from build123d import *

# Parameters (mm, degrees)
BOSS_EXTRUDE1_DEPTH = 5.9944
CUT_EXTRUDE2_REACH  = 7.994


with BuildPart() as part:
    # Sketch1 → Boss-Extrude1 (new body)
    with BuildSketch(Plane.XY):
        Polygon((-3.048, 63.5), (-3.048, 127), (0, 127), (0, 190.5), (-3.048, 190.5), (-3.048, 253.981711342), (59.0804, 253.981711342), (59.0804, 248.012711342), (118.1608, 248.012711342), (118.1608, 253.981711342), (177.2412, 253.981711342), (177.2412, 248.012711342), (236.3216, 248.012711342), (236.3216, 253.981711342), (295.402, 253.981711342), (295.402, 190.481711342), (298.45, 190.481711342), (298.45, 126.981711342), (295.402, 126.981711342), (295.402, 63.5), (298.45, 63.5), (298.45, 0), (0, 0), (0, 63.5), align=None)
    extrude(amount=BOSS_EXTRUDE1_DEPTH)

    # Sketch2 → Cut-Extrude2 (cut, up to next)
    with BuildSketch(Plane.XY.offset(5.9944), mode=Mode.PRIVATE) as cut_extrude2_sk1:
        with BuildLine():
            Line((270.51, 2.54), (270.51, 0))
            Line((270.51, 0), (275.59, 0))
            Line((275.59, 0), (275.59, 2.54))
            ThreePointArc((275.59, 2.54), (273.05, 5.08), (270.51, 2.54))
        make_face()
    cut_extrude2_tool1 = extrude(cut_extrude2_sk1.sketch, amount=-CUT_EXTRUDE2_REACH, mode=Mode.PRIVATE) & part.part
    add(cut_extrude2_tool1.solids().sort_by_distance((273.05, 2.302891, 5.9944))[0], mode=Mode.SUBTRACT)


solid = part.part
The listing builds one solid part. Answer for the finished solid, in the listing's coordinates (mm). A direction names the side the tool comes from. Coordinates: 2 decimals unless noted, no trailing zeros. Write each loop counter-clockwise with the first axis right and the second up, starting at its lowest first coordinate (ties: lowest second). Pieces come first, ordered by that corner, then holes. Notation, with made-up numbers: M 25,13.25 L 51,13.25 A16 cw 51,25.25 Z; hole C 23,71.5 d8. An arc over 180 degrees is marked long. Put each result on its own line as item: value. Start each with the question number.
1. Consider line 1 (X direction, y = 221, z = 1); line 2 (X direction, y = 187.5, z = 2.25); line 3 (Y direction, x = 273, z = 5.45). Determine where each line is inside the solid, lowest interval first. Write a range as from..to.
2. Which of the six approach directions +Z, -Z, +X, -X, +Y, -Y give full straight-line access (tool end or side, diameter ignored) to faces 1 (the flat face through (0, 31, 3)), 2 (the flat face through (0, 158, 3)), 3 (the flat face through (88, 248.013, 3)), 4 (the flat face through (295.402, 223, 3))?
3. A cutting plane is placed at A-A on z = 3.35. Write down the section's boundary in (x, y), then the cut area to 3 significant figures.
4. For a pull along X with two mould halves and no side action, classify faces 5 (the flat face through (298.45, 159, 3)), 6 (the flat face through (59.08, 251, 3)), 7 (the flat face through (287, 0, 3)) as pulls with the +X half, pulls with the -X half, needs draft (parallel to the pull), parting line crosses it, or undercut.
5. A cutting plane is placed at B-B on x = 195. Write down the section's boundary in (y, z).
6. Flat-ended cylindrical pins translate along their axes: P1, Ø1.5, axis at x = 297.5, z = 4, coming from the +Y side; P2, Ø3, axis at y = 232, z = 2.5, coming from the +X side; P3, Ø3.5, axis at x = -1.5, z = 4.5, coming from the -Y side; P4, Ø3, axis at y = 1.5, z = 2, coming from the -X side. Find the tip coordinate at first contact, or state that the pin passes through.
Resolved:
1. line 1: x = -3.05..295.4
1. line 2: x = 0..298.45
1. line 3: y = 5.08..253.98
2. face 1: +Z, -Z, -X, -Y
2. face 2: +Z, -Z, -X
2. face 3: +Z, -Z, +Y
2. face 4: +Z, -Z, +X, +Y
3. outline: M -3.05,63.5 L 0,63.5 L 0,0 L 270.51,0 L 270.51,2.54 A2.54 cw 275.59,2.54 L 275.59,0 L 298.45,0 L 298.45,63.5 L 295.4,63.5 L 295.4,126.98 L 298.45,126.98 L 298.45,190.48 L 295.4,190.48 L 295.4,253.98 L 236.32,253.98 L 236.32,248.01 L 177.24,248.01 L 177.24,253.98 L 118.16,253.98 L 118.16,248.01 L 59.08,248.01 L 59.08,253.98 L -3.05,253.98 L -3.05,190.5 L 0,190.5 L 0,127 L -3.05,127 Z
3. area: 75,100 mm2
4. face 5: pulls with the +X half
4. face 6: undercut
4. face 7: needs draft
5. outline: M 0,0 L 248.01,0 L 248.01,5.99 L 0,5.99 Z
6. P1: stops at y = 190.48
6. P2: stops at x = 295.4
6. P3: stops at y = 0
6. P4: stops at x = 0
